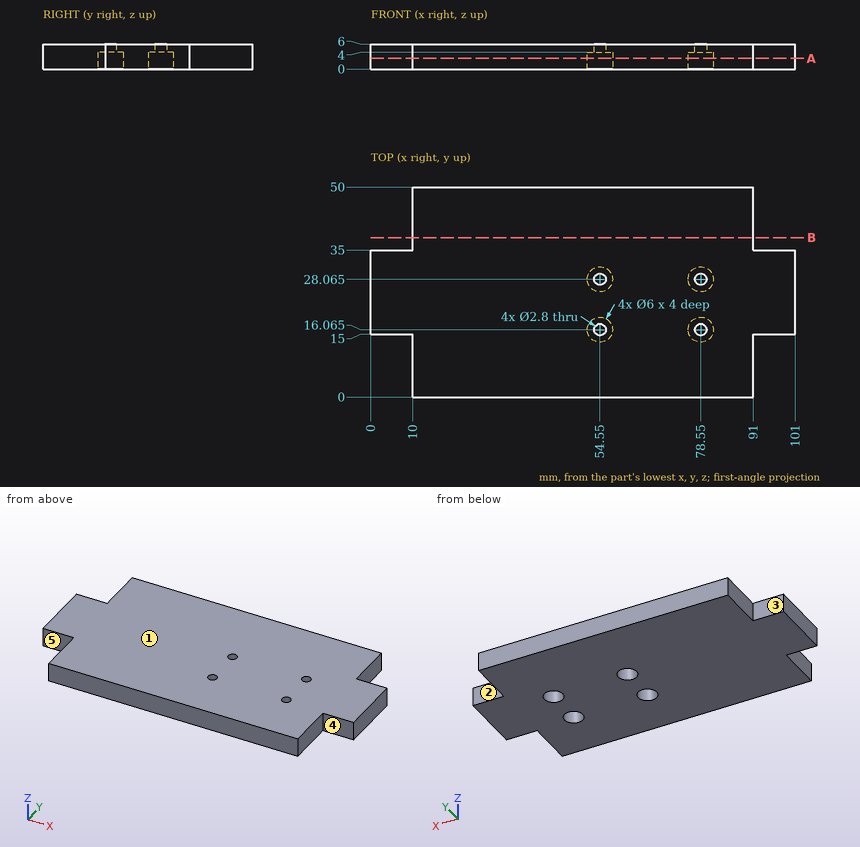
Answer from the drawing. Dimensions are ordinates in mm from the lowest x, y and z of the part. A direction names the side the tool comes from. Give positions to 0.01 mm unless a question says otherwise; leave off trailing zeros. Order: outer loops, then holes, each group sorted by start corner. A loop starts at its lowest first (then second) coordinate and runs counter-clockwise, first axis right, second up. Notation, with made-up numbers: (38.5, -17) -> (85.5, -17) arc R19 ccw to (85.5, -4) -> close; hole circle Ø5 at (-17.5, 81). An arc over 180 degrees is marked (long way). Answer as a JSON object with one key per item and string values. Group by question number.
1. Section A-A on z = 2.55 is taken. Count the separate pieces of the cut face and the enclosed holes in it, plus the area to 3 significant figures.
2. Consider line 1 along Y through (x, z) = (55, 0.55); line 2 along X through (y, z) = (45.5, 5.1); line 3 along Y through (x, z) = (96, 4). Determine where each line is inside the solid, lowest interval first. Write a range as [from, to].
3. Flat-ended cylindrical pins translate along their axes: pin 1 Ø3 at (y, z) = (43, 2) entering from +X; pin 2 Ø1.8 at (x, z) = (95, 3) entering from -Y; pin 3 Ø5 at (x, y) = (54.55, 16.07) entering from -Z. Find the tip coordinate at first contact, or state that the pin passes through.
4. Section B-B on y = 38 is taken. Determine the outline of the cut face in (x, z).
5. A tool of negligible diameter and unlimited length cuts with its end or side. For the marked faces 1, 2, 3, 4 and 5, from which of +Z, -Z, +X, -X, +Y, -Y can it reach the whole face along a straight path? Write none if from no direction.
Result sheet:
{
 "1": {"separate pieces": "1", "enclosed holes": "4", "area": "4,340 mm^2"},
 "2": {"line 1": "y = [0, 13.1], [19.03, 25.1], [31.03, 50]", "line 2": "x = [10, 91]", "line 3": "y = [15, 35]"},
 "3": {"pin 1": "stops at x = 91", "pin 2": "stops at y = 15", "pin 3": "stops at z = 4"},
 "4": {"outline": "(10, 0) -> (91, 0) -> (91, 6) -> (10, 6) -> close"},
 "5": {"face 1": "+Z, +X, -X, +Y, -Y", "face 2": "+Z, -Z, +X, +Y", "face 3": "+Z, -Z, -X, +Y", "face 4": "+Z, -Z, +X, -Y", "face 5": "+Z, -Z, -X, -Y"}
}
